```python
from build123d import *

# Parameters (mm, degrees)
SKETCH1_W           = 54
SKETCH1_H           = 54
SKETCH1_W_2         = 50
SKETCH1_H_2         = 50
BOSS_EXTRUDE1_DEPTH = 75
SKETCH2_R           = 3
CUT_EXTRUDE1_DEPTH  = 25
SKETCH3_R           = 3
CUT_EXTRUDE2_DEPTH  = 25


with BuildPart() as part:
    # Sketch1 → Boss-Extrude1 (new, symmetric)
    with BuildSketch(Plane(origin=(0, 0, 0), x_dir=(0, 0, -1), z_dir=(1, 0, 0))):
        Rectangle(SKETCH1_W, SKETCH1_H)
        Rectangle(SKETCH1_W_2, SKETCH1_H_2, mode=Mode.SUBTRACT)
    extrude(amount=BOSS_EXTRUDE1_DEPTH, both=True)

    # Sketch2 → Cut-Extrude1 (cut)
    with BuildSketch(Plane(origin=(0, 27, 0), x_dir=(1, 0, 0), z_dir=(0, 1, 0))):
        with Locations(Location((-60, 15, 0), (0, 0, 270))):
            Circle(SKETCH2_R)
        with Locations(Location((-60, -15, 0), (0, 0, 270))):
            Circle(SKETCH2_R)
        with Locations(Location((60, 15, 0), (0, 0, 270))):
            Circle(SKETCH2_R)
        with Locations(Location((60, -15, 0), (0, 0, 270))):
            Circle(SKETCH2_R)
        with Locations(Location((-40, -15, 0), (0, 0, 270))):
            Circle(SKETCH2_R)
        with Locations(Location((-40, 15, 0), (0, 0, 270))):
            Circle(SKETCH2_R)
        with Locations(Location((40, -15, 0), (0, 0, 90))):
            Circle(SKETCH2_R)
        with Locations(Location((40, 15, 0), (0, 0, 90))):
            Circle(SKETCH2_R)
    extrude(amount=-CUT_EXTRUDE1_DEPTH, mode=Mode.SUBTRACT)

    # Sketch3 → Cut-Extrude2 (cut)
    with BuildSketch(Plane(origin=(0, 27, 0), x_dir=(1, 0, 0), z_dir=(0, 1, 0))):
        with Locations(Location((-10, 0, 0), (0, 0, 270))):
            Circle(SKETCH3_R)
        with Locations(Location((10, 0, 0), (0, 0, 270))):
            Circle(SKETCH3_R)
    extrude(amount=-CUT_EXTRUDE2_DEPTH, mode=Mode.SUBTRACT)


solid = part.part
```
Geometry: final body of the model. Coordinates: model frame, mm. A direction names the side the tool comes from. Round coordinates to 2 decimals unless told otherwise and drop trailing zeros. Write each loop counter-clockwise with the first axis right and the second up, starting at its lowest first coordinate (ties: lowest second). Pieces come first, ordered by that corner, then holes.
Item 1: Section query A-A (z = -15). Return loops of the section in (x, y), plus the area to 3 significant figures.
Item 2: Material intervals for L1, parallel to Z at x = 40, y = 26.4; L2, parallel to X at y = 26, z = 0; L3, parallel to X at y = 25.4, z = 15, sorted ascending.
Item 3: Mould query, pull axis Z, two halves, no side actions, for faces 4 (the face through (1, 0, -27)), 5 (the face through (37.97, 26.01, -12.79)), 6 (the face through (62.03, 26.01, -17.21)), 7 (the face through (75, -26, 2)). Classes: +Z half, -Z half, draft (parallel to the pull), parting line (faces both ways), or undercut.
Item 4: Set-up query: faces 1 (the face through (10.9, 26.01, 2.86)), 2 (the face through (1, 0, 27)), 3 (the face through (1, 0, 25)). Return all of +Z, -Z, +X, -X, +Y, -Y with unobstructed straight access to the full face (end or side cutting, diameter ignored); none if empty.
Item 5: Section query C-C (y = 19). Return loops of the section in (x, z).
Item 6: Section query B-B (x = 60). Return loops of the section in (y, z), plus the area to 3 significant figures.
Item 7: Pin query (flat end, axial travel): P1, Ø12, axis at y = -15.5, z = 1, coming from the -X side; P2, Ø5.5, axis at x = -40, z = 15, coming from the +Y side. Return the tip coordinate at first contact, or that it passes through.
Item 8: Section query D-D (z = 0). Return loops of the section in (x, y), plus the area to 3 significant figures.
Completed:
1. outline: (-75, -27) - (75, -27) - (75, -25) - (-75, -25) - close; (-75, 25) - (-63, 25) - (-63, 27) - (-75, 27) - close; (-57, 25) - (-43, 25) - (-43, 27) - (-57, 27) - close; (-37, 25) - (37, 25) - (37, 27) - (-37, 27) - close; (43, 25) - (57, 25) - (57, 27) - (43, 27) - close; (63, 25) - (75, 25) - (75, 27) - (63, 27) - close
1. area: 552 mm2
2. L1: z = -27 to -18, -12 to 12, 18 to 27
2. L2: x = -75 to -13, -7 to 7, 13 to 75
2. L3: x = -75 to -63, -57 to -43, -37 to 37, 43 to 57, 63 to 75
3. face 4: -Z half
3. face 5: undercut
3. face 6: undercut
3. face 7: draft
4. face 1: +Y
4. face 2: +Z, +X, -X, +Y, -Y
4. face 3: +X, -X
5. outline: (-75, -27) - (75, -27) - (75, -25) - (-75, -25) - close; (-75, 25) - (75, 25) - (75, 27) - (-75, 27) - close
6. outline: (-27, -27) - (27, -27) - (27, -18) - (25, -18) - (25, -25) - (-25, -25) - (-25, 25) - (25, 25) - (25, 18) - (27, 18) - (27, 27) - (-27, 27) - close; (25, -12) - (27, -12) - (27, 12) - (25, 12) - close
6. area: 392 mm2
7. P1: passes through
7. P2: stops at y = -25
8. outline: (-75, -27) - (75, -27) - (75, -25) - (-75, -25) - close; (-75, 25) - (-13, 25) - (-13, 27) - (-75, 27) - close; (-7, 25) - (7, 25) - (7, 27) - (-7, 27) - close; (13, 25) - (75, 25) - (75, 27) - (13, 27) - close
8. area: 576 mm2
